```python
from build123d import *

# Parameters (mm, degrees)
SKETCH1_R               = 2
BOSS_EXTRUDE1_DEPTH     = 33.3375
SKETCH2_W               = 0.508
SKETCH2_H               = 0.381
CUT_EXTRUDE1_DEPTH      = 34.457269856
CUT_EXTRUDE1_DEPTH_BACK = 34.457269856
SKETCH3_W               = 2.54
SKETCH3_H               = 1.27


with BuildPart() as part:
    # Sketch1 → Boss-Extrude1 (new, symmetric)
    with BuildSketch(Plane.XY):
        Circle(SKETCH1_R)
    extrude(amount=BOSS_EXTRUDE1_DEPTH, both=True)

    # Sketch2 → Cut-Revolve1 (revolve, cut)
    with BuildSketch(Plane(origin=(0, 0, 0), x_dir=(0, 0, -1), z_dir=(1, 0, 0)), mode=Mode.PRIVATE) as cut_revolve1_sk:
        with Locations((-31.46425, 1.8095)):
            Rectangle(SKETCH2_W, SKETCH2_H)
    revolve(cut_revolve1_sk.sketch.rotate(Axis((0, 0, 33.3375), (0, 0, -1)), 90), axis=Axis((0, 0, 33.3375), (0, 0, -1)), mode=Mode.SUBTRACT)

    # Sketch3 → Cut-Extrude1 (cut, two sides: drawn at the far end of the back side and taken through both)
    with BuildSketch(Plane(origin=(0, 0, 0), x_dir=(0, 0, -1), z_dir=(1, 0, 0)).offset(-CUT_EXTRUDE1_DEPTH_BACK)):
        with Locations((32.0675, -1.365)):
            Rectangle(SKETCH3_W, SKETCH3_H)
    extrude(amount=CUT_EXTRUDE1_DEPTH + CUT_EXTRUDE1_DEPTH_BACK, mode=Mode.SUBTRACT)


solid = part.part
```
The model under review builds one solid part; all positions refer to its coordinate system, in mm. A direction names the side the tool comes from. Round coordinates to 2 decimals unless told otherwise and drop trailing zeros. Write each loop counter-clockwise with the first axis right and the second up, starting at its lowest first coordinate (ties: lowest second). Pieces come first, ordered by that corner, then holes. Notation, with made-up numbers: (61.5, -12.75) - (87.5, -12.75) arc R23 ccw to (87.5, -2.75) - close; hole circle Ø8 at (4, 84). An arc over 180 degrees is marked (long way). Answer as CSV lines item,"result". Start each with the question number.
(1) To check wall thickness, follow line 1 (Z direction, x = -0.15, y = 1.8); line 2 (Z direction, x = -1.4, y = -1.05); line 3 (Z direction, x = 0.7, y = -1.3). State the ranges of each line that lie inside material, in increasing order.
(2) We need section C-C on z = -22.5. State the section outline as (x, y) points, plus the area to 3 significant figures.
(3) For faces 1 (the flat face through (0, -1, -30.798)), 2 (the cylindrical face through (0, -2, 33)), list the 3-axis set-ups (+Z, -Z, +X, -X, +Y, -Y) from which the entire face can be reached by the end or side of a thin tool; tool diameter is ignored.
(4) Draft analysis for pull direction Z (two halves, no side actions). For faces 3 (the flat face through (0, 0, -33.338)), 4 (the flat face through (0, 0, 33.338)), 5 (the cylindrical face through (-0.35, 1.58, 31.46)), state which applies: pulls with the +Z half, pulls with the -Z half, needs draft (parallel to the pull), parting line crosses it, or undercut.
(5) We need section A-A on x = 0.4. State the section outline as (y, z) points.
(6) We need section B-B on y = 1.05. State the section outline as (x, z) points, plus the area to 3 significant figures.
Worked answers:
1,line 1,"-33.34 to 31.21, 31.72 to 33.34"
1,line 2,"-30.8 to 31.21, 31.72 to 33.34"
1,line 3,"-30.8 to 33.34"
2,outline,"circle Ø4 at (0, 0)"
2,area,"12.6 mm²"
3,face 1,"-Z, +X, -X, -Y"
3,face 2,"+Z, -Z"
4,face 3,"pulls with the -Z half"
4,face 4,"pulls with the +Z half"
4,face 5,"undercut"
5,outline,"(-1.96, -30.8) - (-0.73, -30.8) - (-0.73, -33.34) - (1.96, -33.34) - (1.96, 31.21) - (1.57, 31.21) - (1.57, 31.72) - (1.96, 31.72) - (1.96, 33.34) - (-1.96, 33.34) - (-1.96, 31.72) - (-1.57, 31.72) - (-1.57, 31.21) - (-1.96, 31.21) - close"
6,outline,"(-1.7, -33.34) - (1.7, -33.34) - (1.7, 31.21) - (1.23, 31.21) - (1.23, 31.72) - (1.7, 31.72) - (1.7, 33.34) - (-1.7, 33.34) - (-1.7, 31.72) - (-1.23, 31.72) - (-1.23, 31.21) - (-1.7, 31.21) - close"
6,area,"227 mm²"
